Verification items for the finished model (mm, model axes). A direction names the side the tool comes from. Round coordinates to 2 decimals unless told otherwise and drop trailing zeros. Loops run counter-clockwise (first coordinate to the right, second up) from the corner with the lowest first, then second, coordinate; pieces in that order, holes last. Notation, with made-up numbers: (34, -35.75) -> (68, -35.75) arc R21 ccw to (68, -16.75) -> close; hole circle Ø5 at (-18.5, 39.25). An arc over 180 degrees is marked (long way). Use a Markdown table: item, result. Add a question column.
```python
from build123d import *

# Parameters (mm, degrees)
SKETCH1_R                   = 12
BOSS_EXTRUDE1_DEPTH         = 3
TAP_DRILL_FOR_M3_TAP1_D     = 2.5
TAP_DRILL_FOR_M3_TAP1_DEPTH = 5
TAP_DRILL_FOR_M3_TAP1_TIP   = 0.751075774
TAP_DRILL_FOR_M6_TAP1_D     = 5
TAP_DRILL_FOR_M6_TAP1_DEPTH = 5
TAP_DRILL_FOR_M6_TAP1_TIP   = 1.502151548
FILLET1_R                   = 2
TAP_DRILL_FOR_M2_TAP1_D     = 1.6
TAP_DRILL_FOR_M2_TAP1_DEPTH = 5
TAP_DRILL_FOR_M2_TAP1_TIP   = 0.480688495
CUT_EXTRUDE1_DEPTH          = 10


with BuildPart() as part:
    # Sketch1 → Boss-Extrude1 (new body)
    with BuildSketch(Plane.XY):
        Polygon((18.05, -51.655), (18.05, -21.05), (21.05, -18.05), (21.05, 18.05), (18.05, 21.05), (-18.05, 21.05), (-21.05, 18.05), (-21.05, -18.05), (-18.05, -21.05), (-18.05, -51.655), align=None)
        Circle(SKETCH1_R, mode=Mode.SUBTRACT)
    extrude(amount=BOSS_EXTRUDE1_DEPTH)

    # Tap Drill for M3 Tap1
    with Locations(Plane.XY.offset(3)):
        with Locations((-15.5, 15.5), (15.5, 15.5), (-15.5, -15.5), (15.5, -15.5)):
            Hole(TAP_DRILL_FOR_M3_TAP1_D / 2, depth=TAP_DRILL_FOR_M3_TAP1_DEPTH)
            with Locations((0, 0, -(TAP_DRILL_FOR_M3_TAP1_DEPTH + TAP_DRILL_FOR_M3_TAP1_TIP / 2))):  # 118° drill point
                Cone(0, TAP_DRILL_FOR_M3_TAP1_D / 2, TAP_DRILL_FOR_M3_TAP1_TIP, mode=Mode.SUBTRACT)

    # Tap Drill for M6 Tap1
    with Locations(Plane.XY.offset(3)):
        with Locations((-12, -36.655), (12, -36.655)):
            Hole(TAP_DRILL_FOR_M6_TAP1_D / 2, depth=TAP_DRILL_FOR_M6_TAP1_DEPTH)
            with Locations((0, 0, -(TAP_DRILL_FOR_M6_TAP1_DEPTH + TAP_DRILL_FOR_M6_TAP1_TIP / 2))):  # 118° drill point
                Cone(0, TAP_DRILL_FOR_M6_TAP1_D / 2, TAP_DRILL_FOR_M6_TAP1_TIP, mode=Mode.SUBTRACT)

    # Fillet1
    fillet1_edges = [part.edges().sort_by_distance(p)[0] for p in [
        (18.05, -21.05, 1.5),
        (18.05, -51.655, 1.5),
        (-18.05, -51.655, 1.5),
        (-18.05, -21.05, 1.5),
    ]]
    fillet(fillet1_edges, radius=FILLET1_R)

    # Tap Drill for M2 Tap1
    with Locations(Plane.XY.offset(3)):
        with Locations((10.52945603, -21.86131015), (10.52945603, -28.56131015)):
            Hole(TAP_DRILL_FOR_M2_TAP1_D / 2, depth=TAP_DRILL_FOR_M2_TAP1_DEPTH)
            with Locations((0, 0, -(TAP_DRILL_FOR_M2_TAP1_DEPTH + TAP_DRILL_FOR_M2_TAP1_TIP / 2))):  # 118° drill point
                Cone(0, TAP_DRILL_FOR_M2_TAP1_D / 2, TAP_DRILL_FOR_M2_TAP1_TIP, mode=Mode.SUBTRACT)

    # Sketch8 → Cut-Extrude1 (cut)
    with BuildSketch(Plane(origin=(0, 0, 0), x_dir=(-1, 0, 0), z_dir=(0, 0, -1))):
        with BuildLine():
            Line((-0.855282685, -36.386266358), (2.992061815, -30.914487513))
            ThreePointArc((2.992061815, -30.914487513), (2.60653362, -28.702773131), (0.394819237, -29.088301326))
            Line((0.394819237, -29.088301326), (-0.119454204, -29.819712442))
            Line((-0.119454204, -29.819712442), (-1.013815468, -28.896697877))
            ThreePointArc((-1.013815468, -28.896697877), (-3.258600516, -28.861305914), (-3.293992479, -31.106090962))
            Line((-3.293992479, -31.106090962), (-1.978516355, -32.463711947))
            Line((-1.978516355, -32.463711947), (-3.452525263, -34.56008017))
            ThreePointArc((-3.452525263, -34.56008017), (-3.066997067, -36.771794553), (-0.855282685, -36.386266358))
        make_face()
    extrude(amount=-CUT_EXTRUDE1_DEPTH, mode=Mode.SUBTRACT)


solid = part.part
```
1) Release check for a two-part mould opening along X. For faces 1 (the face through (10.703, -29.342, 1.479)), 2 (the face through (0, -51.655, 1)), 3 (the face through (17.48, -51.054, 1.521)), 4 (the face through (-11.99, 0.53, 1.48)) record: released by +X, released by -X, zero draft, split by the parting line, or undercut.
2) Sectioned sample at D-D on z = 1.15. State how many separate pieces and enclosed holes the cut face has, then the cut area to 3 significant figures.
3) Go/stop test with flat-tipped pins: pin 1 (2 mm diameter, centred on x = -15.5, y = 15.5, fed in from -Z); pin 2 (1.5 mm diameter, centred on y = -30.5, z = 1.5, fed in from -X). Record where each tip stops, or that it passes through.
4) Access from +Z, -Z, +X, -X, +Y, -Y to the whole of each face (thin tool, end or side, straight path). Record for faces 5 (the face through (-18.05, -36, 1)), 6 (the face through (18.05, -36, 1)), 7 (the face through (2.645, -31.775, 1.479)).
5) Thickness scan on line 1 (Y direction, x = -15.5, z = 1.55) (3 decimals); line 2 (Y direction, x = 0, z = 1.7) (3 decimals); line 3 (Y direction, x = 3.5, z = 0.45) (3 decimals). Record the ranges inside material, lowest first.
6) Sectioned sample at C-C on y = 4. Enter the section's corners in (x, z).
7) Sectioned sample at A-A on y = -15.5. Enter the section's corners in (x, z), then the cut area to 3 significant figures.
8) Sectioned sample at B-B on x = 5.5. Enter the section's corners in (y, z) (3 decimals).
Geometry results:
| question | item | result |
|---|---|---|
| 1 | face 1 | undercut |
| 1 | face 2 | zero draft |
| 1 | face 3 | released by +X |
| 1 | face 4 | undercut |
| 2 | separate pieces | 1 |
| 2 | enclosed holes | 10 |
| 2 | area | 2,300 mm^2 |
| 3 | pin 1 | through |
| 3 | pin 2 | x = -18.05 |
| 4 | face 5 | +Z, -Z, -X, -Y |
| 4 | face 6 | +Z, -Z, +X, -Y |
| 4 | face 7 | +Z, -Z |
| 5 | line 1 | -51.655 to -16.75, -14.25 to 14.25, 16.75 to 21.05 |
| 5 | line 2 | -51.655 to -35.17, -29.65 to -12, 12 to 21.05 |
| 5 | line 3 | -51.655 to -36.315, -34.632 to -30.843, -29.16 to -11.478, 11.478 to 21.05 |
| 6 | outline | (-21.05, 0) -> (-11.31, 0) -> (-11.31, 3) -> (-21.05, 3) -> close; (11.31, 0) -> (21.05, 0) -> (21.05, 3) -> (11.31, 3) -> close |
| 7 | outline | (-21.05, 0) -> (-16.75, 0) -> (-16.75, 3) -> (-21.05, 3) -> close; (-14.25, 0) -> (14.25, 0) -> (14.25, 3) -> (-14.25, 3) -> close; (16.75, 0) -> (21.05, 0) -> (21.05, 3) -> (16.75, 3) -> close |
| 7 | area | 111 mm^2 |
| 8 | outline | (-51.655, 0) -> (-10.665, 0) -> (-10.665, 3) -> (-51.655, 3) -> close; (10.665, 0) -> (21.05, 0) -> (21.05, 3) -> (10.665, 3) -> close |
